Build history of the part. All positions in model axes, mm. Face numbers are marked on the shaded views. A direction names the side the tool comes from. Give positions to 0.01 mm unless a question says otherwise; leave off trailing zeros. Order: outer loops, then holes, each group sorted by start corner. A loop starts at its lowest first (then second) coordinate and runs counter-clockwise, first axis right, second up. Notation, with made-up numbers: (56, 39) - (100, 39) arc R17 ccw to (100, 48) - close; hole circle Ø6 at (73.25, -31). An arc over 180 degrees is marked (long way). Use a Markdown table: item, result. Add a question column.
(1) Slice it at C-C (x = 62.5). Write the cut outline in (y, z).
(2) Slice it at B-B (y = 16.5). Write the cut outline in (x, z).
(3) Wall check: line 1 (X direction, y = 42, z = 3.5); line 2 (Y direction, x = 62.5, z = 3.25); line 3 (X direction, y = 42, z = 0.5). Give the ranges that are in metal, low to high.
(4) Slice it at D-D (y = 53.5). Write the cut outline in (x, z).
(5) Slice it at A-A (x = 42.5). Write the cut outline in (y, z), then the cut area to 3 significant figures.
(6) Which spindle directions (+Z, -Z, +X, -X, +Y, -Y) get a long thin tool onto all of the face, cutting with end or side? Do the marked faces 1 and 2. Say none if no direction does.
(7) Flat gauge pins, fed straight in: pin 1 (4 mm diameter, centred on x = 70, y = 22, fed in from -Z); pin 2 (2.5 mm diameter, centred on y = 70.5, z = 5, fed in from +X); pin 3 (1 mm diameter, centred on x = 106.5, z = 1.5, fed in from -Y). Where does each tip first touch, or does it go through?
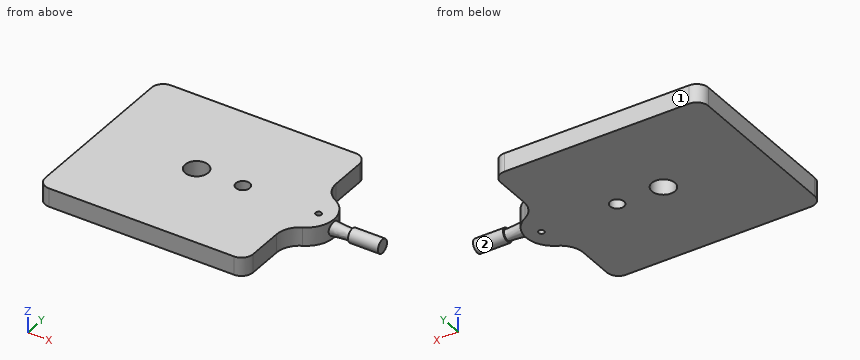
from build123d import *

# Parameters (mm, degrees)
SKETCH1_R                = 5
BOSS_EXTRUDE1_DEPTH      = 8
BOSS_EXTRUDE2_DEPTH      = 10
BOSS_EXTRUDE2_DEPTH_BACK = 3
SKETCH4_R                = 2.970033329
FILLET6_R                = 5
SKETCH5_R                = 1.25
CUT_EXTRUDE2_DEPTH       = 10
SKETCH6_R                = 3
CUT_EXTRUDE3_DEPTH       = 10


with BuildPart() as part:
    # Sketch1 → Boss-Extrude1 (new body)
    with BuildSketch(Plane.XY):
        with BuildLine():
            Line((0, 25.404082058), (0, 80))
            Line((0, 80), (90, 80))
            Line((90, 80), (90, 59.595917942))
            ThreePointArc((90, 59.595917942), (91.471971346, 54.373588264), (95.454545455, 50.688682514))
            ThreePointArc((95.454545455, 50.688682514), (102, 40), (95.454545455, 29.311317486))
            ThreePointArc((95.454545455, 29.311317486), (91.471971346, 25.626411736), (90, 20.404082058))
            Line((90, 20.404082058), (90, 0))
            Line((90, 0), (0, 0))
            Line((0, 0), (0, 25.404082058))
        make_face()
        with Locations((42.5, 40)):
            Circle(SKETCH1_R, mode=Mode.SUBTRACT)
    extrude(amount=BOSS_EXTRUDE1_DEPTH)

    # Loft1: read off the stored shape, not the designer's step
    # Loft1: loft between two sections, ruled curve by curve
    loft1_from = [
        Edge.make_bspline([(98, 43.257575322, 2.799379564), (98, 45.658816193, 9.314530208), (98, 39.143665549, 11.715771079), (98, 36.742424678, 5.200620436), (98, 34.341183807, -1.314530208), (98, 40.856334451, -3.715771079), (98, 43.257575322, 2.799379564)], [0, 0, 0, 0, 0.5, 0.5, 0.5, 1, 1, 1, 1], 3, [1, 0.333333333, 0.333333333, 1, 0.333333333, 0.333333333, 1]),
    ]
    loft1_to = [
        Edge.make_bspline([(113, 40.429483248, 1.709498759), (113, 45.010485729, 2.568465255), (113, 44.151519233, 7.149467737), (113, 39.570516752, 6.290501241), (113, 34.989514271, 5.431534745), (113, 35.848480767, 0.850532263), (113, 40.429483248, 1.709498759)], [0, 0, 0, 0, 0.5, 0.5, 0.5, 1, 1, 1, 1], 3, [1, 0.333333333, 0.333333333, 1, 0.333333333, 0.333333333, 1]),
    ]
    loft1 = Solid(Shell([*[Face.make_surface_from_curves(loft1_from[k], loft1_to[k]) for k in range(1)], Face(Wire(loft1_from)), Face(Wire(loft1_to))]))
    add(loft1)

    # Sketch4 → Boss-Extrude2 (add, two sides: drawn at the far end of the back side and taken through both)
    with BuildSketch(Plane(origin=(113, 0, 0), x_dir=(0, 0, -1), z_dir=(1, 0, 0)).offset(-BOSS_EXTRUDE2_DEPTH_BACK)):
        with Locations((-4, 40)):
            Circle(SKETCH4_R)
    extrude(amount=BOSS_EXTRUDE2_DEPTH + BOSS_EXTRUDE2_DEPTH_BACK)

    # Fillet6
    fillet6_edges = [part.edges().sort_by_distance(p)[0] for p in [
        (0, 80, 4),
        (90, 80, 4),
        (90, 0, 4),
        (0, 0, 4),
    ]]
    fillet(fillet6_edges, radius=FILLET6_R)

    # Sketch5 → Cut-Extrude2 (cut)
    with BuildSketch(Plane.XY.offset(8)):
        with Locations((95.34, 40)):
            Circle(SKETCH5_R)
    extrude(amount=-CUT_EXTRUDE2_DEPTH, mode=Mode.SUBTRACT)

    # Sketch6 → Cut-Extrude3 (cut)
    with BuildSketch(Plane.XY.offset(8)):
        with Locations((62.5, 40.062959469)):
            Circle(SKETCH6_R)
    extrude(amount=-CUT_EXTRUDE3_DEPTH, mode=Mode.SUBTRACT)


solid = part.part
Solution:
| question | item | result |
|---|---|---|
| 1 | outline | (0, 0) - (37.06, 0) - (37.06, 8) - (0, 8) - close; (43.06, 0) - (80, 0) - (80, 8) - (43.06, 8) - close |
| 2 | outline | (0, 0) - (90, 0) - (90, 8) - (0, 8) - close |
| 3 | line 1 | 0 to 37.92, 47.08 to 60.21, 64.79 to 123 |
| 3 | line 2 | 0 to 37.06, 43.06 to 80 |
| 3 | line 3 | 0 to 37.92, 47.08 to 60.21, 64.79 to 101.83 |
| 4 | outline | (0, 0) - (92.07, 0) - (92.07, 8) - (0, 8) - close |
| 5 | outline | (0, 0) - (35, 0) - (35, 8) - (0, 8) - close; (45, 0) - (80, 0) - (80, 8) - (45, 8) - close |
| 5 | area | 560 mm2 |
| 6 | face 1 | +Z, -Z, +X, -X, +Y |
| 6 | face 2 | +X |
| 7 | pin 1 | z = 0 |
| 7 | pin 2 | x = 90 |
| 7 | pin 3 | y = 38.57 |
